Autodesk Inventor part; units mm, degrees
ref_plane "Work Plane1" through (1.0182, 4.3839, -28.4508) normal (0, 0, 1) x (1, 0, 0)
ref_plane "YZ Plane" through (0, 0, 0) normal (1, 0, 0) x (0, 1, 0)
ref_plane "XZ Plane" through (0, 0, 0) normal (0, 1, 0) x (-1, 0, 0)
ref_plane "Work Plane1" through (1.0182, 4.3839, -28.4508) normal (0, 0, 1) x (1, 0, 0)
sketch "Sketch4" plane through (1.0182, 4.3839, -28.4508) normal (0, 0, 1) x (1, 0, 0)
  arc A0 (100, 130) -> (90, 140) centre (90, 130) ccw construction
  line L0 (-90, 140) -> (90, 140) construction
  arc A1 (-90, 140) -> (-100, 130) centre (-90, 130) ccw construction
  line L1 (-100, 110) -> (-100, 130) construction
  arc A2 (-110, 100) -> (-100, 110) centre (-110, 110) ccw construction
  line L2 (-130, 100) -> (-110, 100) construction
  arc A3 (-130, 100) -> (-140, 90) centre (-130, 90) ccw construction
  line L3 (-140, -90) -> (-140, 90) construction
  arc A4 (-140, -90) -> (-130, -100) centre (-130, -90) ccw construction
  line L4 (-110, -100) -> (-130, -100) construction
  arc A5 (-100, -110) -> (-110, -100) centre (-110, -110) ccw construction
  line L5 (-100, -130) -> (-100, -110) construction
  arc A6 (-100, -130) -> (-90, -140) centre (-90, -130) ccw construction
  line L6 (90, -140) -> (-90, -140) construction
  arc A7 (90, -140) -> (100, -130) centre (90, -130) ccw construction
  line L7 (100, -110) -> (100, -130) construction
  arc A8 (110, -100) -> (100, -110) centre (110, -110) ccw construction
  line L8 (130, -100) -> (110, -100) construction
  arc A9 (130, -100) -> (140, -90) centre (130, -90) ccw construction
  line L9 (140, 90) -> (140, -90) construction
  arc A10 (140, 90) -> (130, 100) centre (130, 90) ccw construction
  line L10 (110, 100) -> (130, 100) construction
  arc A11 (100, 110) -> (110, 100) centre (110, 110) ccw construction
  line L11 (100, 130) -> (100, 110) construction
  circle A12 centre (0, 125) radius 3.75 construction
  circle A13 centre (0, -125) radius 3.75 construction
  circle A14 centre (-125, 0) radius 3.75 construction
  circle A15 centre (125, 0) radius 3.75 construction
  arc A16 (98.5, 130) -> (90, 138.5) centre (90, 130) ccw
  line L12 (98.5, 130) -> (98.5, 110)
  arc A17 (98.5, 110) -> (110, 98.5) centre (110, 110) ccw
  line L13 (110, 98.5) -> (130, 98.5)
  arc A18 (138.5, 90) -> (130, 98.5) centre (130, 90) ccw
  line L14 (138.5, 90) -> (138.5, -90)
  arc A19 (130, -98.5) -> (138.5, -90) centre (130, -90) ccw
  line L15 (130, -98.5) -> (110, -98.5)
  arc A20 (110, -98.5) -> (98.5, -110) centre (110, -110) ccw
  line L16 (98.5, -110) -> (98.5, -130)
  arc A21 (90, -138.5) -> (98.5, -130) centre (90, -130) ccw
  line L17 (90, -138.5) -> (-90, -138.5)
  arc A22 (-98.5, -130) -> (-90, -138.5) centre (-90, -130) ccw
  line L18 (-98.5, -130) -> (-98.5, -110)
  arc A23 (-98.5, -110) -> (-110, -98.5) centre (-110, -110) ccw
  line L19 (-110, -98.5) -> (-130, -98.5)
  arc A24 (-138.5, -90) -> (-130, -98.5) centre (-130, -90) ccw
  line L20 (-138.5, -90) -> (-138.5, 90)
  arc A25 (-130, 98.5) -> (-138.5, 90) centre (-130, 90) ccw
  line L21 (-130, 98.5) -> (-110, 98.5)
  arc A26 (-110, 98.5) -> (-98.5, 110) centre (-110, 110) ccw
  line L22 (-98.5, 110) -> (-98.5, 130)
  arc A27 (-90, 138.5) -> (-98.5, 130) centre (-90, 130) ccw
  line L23 (-90, 138.5) -> (90, 138.5)
  line L24 (-125, 0) -> (-113.2017, 0)
  circle A28 centre (2.5, 125) radius 3.75
  circle A29 centre (-122.5, 0) radius 3.75
  circle A30 centre (127.5, 0) radius 3.75
  circle A31 centre (1.5, -125) radius 3.75
  point P0 (-1.0182, -4.3839)
  dimension "d21" = 1.5
  dimension "d22" = 2.5
  dimension "d23" = 2.5
  dimension "d24" = 2.5
  dimension "d25" = 1.5
  dimension "d26" = 7.5
  dimension "d27" = 7.5
  dimension "d28" = 7.5
  dimension "d29" = 7.5
  dimension "d30" = 7.5
extrude "Extrusion3" add sketch "Sketch4" along normal blind 8
sketch "Sketch6" plane through (1.0182, 4.3839, -20.4508) normal (0, 0, 1) x (1, 0, 0)
  arc A0 (98.5, 130) -> (90, 138.5) centre (90, 130) ccw
  line L0 (90, 138.5) -> (-90, 138.5)
  arc A1 (-90, 138.5) -> (-98.5, 130) centre (-90, 130) ccw
  line L1 (-98.5, 130) -> (-98.5, 110)
  arc A2 (-110, 98.5) -> (-98.5, 110) centre (-110, 110) ccw
  line L2 (-110, 98.5) -> (-130, 98.5)
  arc A3 (-130, 98.5) -> (-138.5, 90) centre (-130, 90) ccw
  line L3 (-138.5, 90) -> (-138.5, -90)
  arc A4 (-138.5, -90) -> (-130, -98.5) centre (-130, -90) ccw
  line L4 (-130, -98.5) -> (-110, -98.5)
  arc A5 (-98.5, -110) -> (-110, -98.5) centre (-110, -110) ccw
  line L5 (-98.5, -110) -> (-98.5, -130)
  arc A6 (-98.5, -130) -> (-90, -138.5) centre (-90, -130) ccw
  line L6 (-90, -138.5) -> (90, -138.5)
  arc A7 (90, -138.5) -> (98.5, -130) centre (90, -130) ccw
  line L7 (98.5, -130) -> (98.5, -110)
  arc A8 (110, -98.5) -> (98.5, -110) centre (110, -110) ccw
  line L8 (110, -98.5) -> (130, -98.5)
  arc A9 (130, -98.5) -> (138.5, -90) centre (130, -90) ccw
  line L9 (138.5, -90) -> (138.5, 90)
  arc A10 (138.5, 90) -> (130, 98.5) centre (130, 90) ccw
  line L10 (130, 98.5) -> (110, 98.5)
  arc A11 (98.5, 110) -> (110, 98.5) centre (110, 110) ccw
  line L11 (98.5, 110) -> (98.5, 130)
  circle A12 centre (1.5, -125) radius 3.75
  circle A13 centre (127.5, 0) radius 3.75
  circle A14 centre (-122.5, 0) radius 3.75
  circle A15 centre (2.5, 125) radius 3.75
  point P0 (-1.0182, -4.3839)
equation "\"d27\" = d26"
equation "\"d28\" = d27"
equation "\"d29\" = d28"
equation "\"d30\" = d28"
properties part number "_3DPrint"
Source: CAD feature listing. Evaluate the final solid. Frame: model axes, mm. A direction names the side the tool comes from. Round coordinates to 2 decimals unless told otherwise and drop trailing zeros. Write each loop counter-clockwise with the first axis right and the second up, starting at its lowest first coordinate (ties: lowest second). Pieces come first, ordered by that corner, then holes. Notation, with made-up numbers: (-32.75, -30) - (-27.75, -30) arc R18 cw to (-27.75, 1) - close; hole circle Ø11 at (52, 86). An arc over 180 degrees is marked (long way). Use CSV: the item, a comma, the result in double quotes. Start each with the question number.
(1) Set-up query: faces 5 (the face through (-97.482, 124, -25)), 6 (the face through (99.518, -115, -25)), 7 (the face through (102.98, 106.16, -24.51)). Return all of +Z, -Z, +X, -X, +Y, -Y with unobstructed straight access to the full face (end or side cutting, diameter ignored); none if empty.
(2) First-contact query: pin 1 Ø2.5 at (y, z) = (-113.5, -24) entering from +X; pin 2 Ø2.5 at (y, z) = (121.5, -25.5) entering from -X; pin 3 Ø2.5 at (x, z) = (116.5, -23) entering from -Y. Flat tips, straight axial feed; report the tip coordinate or a pass-through.
(3) Cut plane A-A, the plane z = -26.25. Return loops of the section in (x, y), and give its area (3 significant figures).
(4) Material intervals for probe 1 along X at (y, z) = (-120, -25); probe 2 along Y at (x, z) = (-109.5, -27); probe 3 along Y at (x, z) = (126, -21), sorted ascending. Write a range as [from, to].
(5) Mould query, pull axis X, two halves, no side actions, for faces 1 (the face through (-119, -94.116, -25)), 2 (the face through (-95.058, 140.328, -24.507)), 3 (the face through (124.77, 4.22, -24.51)), 4 (the face through (137.094, -91.56, -24.507)). Classes: pulls with the +X half, pulls with the -X half, needs draft (parallel to the pull), parting line crosses it, or undercut.
Geometry says:
1,face 5,"+Z, -Z, -X, +Y"
1,face 6,"+Z, -Z, +X, -Y"
1,face 7,"+Z, -Z, +X, +Y"
2,pin 1,"x = 99.52"
2,pin 2,"x = -97.48"
2,pin 3,"y = -94.12"
3,outline,"(-137.48, -85.62) arc R8.5 ccw to (-128.98, -94.12) - (-108.98, -94.12) arc R11.5 cw to (-97.48, -105.62) - (-97.48, -125.62) arc R8.5 ccw to (-88.98, -134.12) - (91.02, -134.12) arc R8.5 ccw to (99.52, -125.62) - (99.52, -105.62) arc R11.5 cw to (111.02, -94.12) - (131.02, -94.12) arc R8.5 ccw to (139.52, -85.62) - (139.52, 94.38) arc R8.5 ccw to (131.02, 102.88) - (111.02, 102.88) arc R11.5 cw to (99.52, 114.38) - (99.52, 134.38) arc R8.5 ccw to (91.02, 142.88) - (-88.98, 142.88) arc R8.5 ccw to (-97.48, 134.38) - (-97.48, 114.38) arc R11.5 cw to (-108.98, 102.88) - (-128.98, 102.88) arc R8.5 ccw to (-137.48, 94.38) - close; hole circle Ø7.5 at (-121.48, 4.38); hole circle Ø7.5 at (2.52, -120.62); hole circle Ø7.5 at (3.52, 129.38); hole circle Ø7.5 at (128.52, 4.38)"
3,area,"70,100 mm²"
4,probe 1,"[-97.48, -1.18], [6.22, 99.52]"
4,probe 2,"[-94.12, 102.88]"
4,probe 3,"[-94.12, 1.61], [7.16, 102.88]"
5,face 1,"needs draft"
5,face 2,"pulls with the -X half"
5,face 3,"undercut"
5,face 4,"pulls with the +X half"
